CAD build for the part. Positions are in the model's coordinates, mm. A direction names the side the tool comes from. Coordinates: 2 decimals unless noted, no trailing zeros. Loops run counter-clockwise (first coordinate to the right, second up) from the corner with the lowest first, then second, coordinate; pieces in that order, holes last. Notation, with made-up numbers: (43, 33) -> (64, 33) arc R9 cw to (64, 40) -> close; hole circle Ø5 at (32, 78). An arc over 180 degrees is marked (long way). Write each question's results on one line, items separated by ' | '.
Autodesk Inventor part; units mm, degrees
ref_plane "YZ Plane" through (0, 0, 0) normal (1, 0, 0) x (0, 1, 0)
ref_plane "XZ Plane" through (0, 0, 0) normal (0, 1, 0) x (-1, 0, 0)
ref_plane "XY Plane" through (0, 0, 0) normal (0, 0, 1) x (1, 0, 0)
sketch "Boceto1" plane through (0, 0, 0) normal (0, 1, 0) x (-1, 0, 0)
  circle A0 centre (28.5, 0) radius 1.5
  circle A1 centre (28.5, -8) radius 1.5
  circle A2 centre (28.5, 8) radius 1.5
  circle A3 centre (36.5, 0) radius 1.5
  circle A4 centre (20.5, 0) radius 1.5
  circle A5 centre (28.5, 0) radius 47.5
  line L0 (57, 33) -> (43, 33)
  line L1 (43, 33) -> (43, 30)
  line L2 (35.5, 30) -> (35.5, 33)
  line L3 (35.5, 33) -> (21.5, 33)
  line L4 (21.5, 33) -> (21.5, 30)
  line L5 (14, 30) -> (14, 33)
  line L6 (14, 33) -> (0, 33)
  line L7 (43, 30) -> (57, 30)
  line L8 (21.5, 30) -> (35.5, 30)
  line L9 (14, 30) -> (0, 30)
  line L10 (0, 30) -> (0, 33)
  line L11 (57, 33) -> (57, 30)
  line L12 (35.5, -30) -> (35.5, -33)
  line L13 (21.5, -30) -> (35.5, -30)
  line L14 (35.5, -33) -> (21.5, -33)
  line L15 (21.5, -33) -> (21.5, -30)
  line L16 (57, -33) -> (43, -33)
  line L17 (43, -33) -> (43, -30)
  line L18 (43, -30) -> (57, -30)
  line L19 (14, -30) -> (14, -33)
  line L20 (14, -30) -> (0, -30)
  line L21 (14, -33) -> (0, -33)
  line L22 (0, -30) -> (0, -33)
  line L23 (57, -33) -> (57, -30)
extrude "Extrusión1" add sketch "Boceto1" along normal blind 3
sketch "Boceto2" plane through (-28.5, 0, 0) normal (0, -1, 0) x (1, 0, 0)
  circle A0 centre (0, 0) radius 3.5
  point P0 (28.5, 0)
  dimension "d23" = 7
extrude "Extrusión2" cut sketch "Boceto2" against normal blind 10
sketch "Boceto3" plane through (-28.5, 0, 0) normal (0, -1, 0) x (1, 0, 0)
  circle A0 centre (0, 0) radius 4.5
  point P0 (28.5, 0)
  dimension "d26" = 9
extrude "Extrusión3" cut sketch "Boceto3" against normal blind 10
sketch "Boceto4" plane through (-28.5, 0, 0) normal (0, -1, 0) x (1, 0, 0)
  arc A0 (-36.5, 30) -> (-36.5, -30) centre (0, 0) ccw
  line L0 (-28.5, 30) -> (-28.5, 33)
  line L1 (-36.5, 30) -> (-109.5, 30)
  line L2 (-109.5, 30) -> (-109.5, -30)
  line L3 (-28.5, -33) -> (-28.5, -30)
  line L4 (-109.5, -30) -> (-36.5, -30)
extrude "Extrusión4" add sketch "Boceto4" against normal blind 3
sketch "Boceto5" plane through (0, 3, 0) normal (0, 1, 0) x (1, 0, 0)
  line L0 (-11.1092, 17.1983) -> (-42.6801, 17.1983)
  line L1 (-42.6801, 17.1983) -> (-42.6801, -13.2583)
  line L2 (-42.6801, -13.2583) -> (-11.1092, -13.2583)
  line L3 (-11.1092, -13.2583) -> (-11.1092, 17.1983)
  point P0 (0, 0)
extrude "Extrusión5" add sketch "Boceto5" against normal blind 3
properties part number "base3"
Q1. Pull direction X, two halves, no side cores. Call faces 1 (the flat face through (-29, 1, 33)), 2 (the flat face through (-58, 0, 1)), 3 (the cylindrical face through (18.972, 1.479, -1.634)): +X half, -X half, draft (parallel to the pull), parting line (faces both ways), or undercut.
Results are:
face 1: undercut | face 2: draft | face 3: parting line
Q2. Cut at C-C on x = -48. Write the cut outline in (y, z), and give its area (3 significant figures).
Results are:
outline: (0, -43.31) -> (3, -43.31) -> (3, -33) -> (0, -33) -> close; (0, -30) -> (3, -30) -> (3, 30) -> (0, 30) -> close; (0, 33) -> (3, 33) -> (3, 43.31) -> (0, 43.31) -> close | area: 242 mm^2
Q3. Drop flat-ended pins along their axis: pin 1 (0.9 mm diameter, centred on y = 1.5, z = -32, fed in from +X); pin 2 (1.5 mm diameter, centred on y = 1.5, z = 31.5, fed in from -X); pin 3 (1.5 mm diameter, centred on x = -118, y = 1, fed in from +Z). Give the stop position or say it passes through.
Results are:
pin 1: x = 7.01 | pin 2: x = -64.7 | pin 3: z = 30
Q4. Cut at B-B on y = 1.55. Write the cut outline in (x, z).
Results are:
outline: (-138, -30) -> (-65.33, -30) arc R47.5 ccw (long way) to (-65.33, 30) -> (-138, 30) -> close; hole (-57, -33) -> (-43, -33) -> (-43, -30) -> (-57, -30) -> close; hole (-57, 30) -> (-43, 30) -> (-43, 33) -> (-57, 33) -> close; hole (-35.5, -33) -> (-21.5, -33) -> (-21.5, -30) -> (-35.5, -30) -> close; hole (-35.5, 30) -> (-21.5, 30) -> (-21.5, 33) -> (-35.5, 33) -> close; hole (-14, -33) -> (0, -33) -> (0, -30) -> (-14, -30) -> close; hole (-14, 30) -> (0, 30) -> (0, 33) -> (-14, 33) -> close
Q5. Wall check: L1, parallel to Z at x = -27, y = 1.95; L2, parallel to Z at x = -44.5, y = 0.5; L3, parallel to Z at x = -76.5, y = 1.8. Give the ranges that are in metal, low to high. Write a range as from..to.
Results are:
L1: -47.48..-33, -30..30, 33..47.48 | L2: -44.72..-33, -30..30, 33..44.72 | L3: -30..30
Q6. Cut at D-D on x = -105. Write the cut outline in (y, z), and give its area (3 significant figures).
Results are:
outline: (0, -30) -> (3, -30) -> (3, 30) -> (0, 30) -> close | area: 180 mm^2
Q7. Cut at A-A on x = -28.5. Write the cut outline in (y, z).
Results are:
outline: (0, -47.5) -> (3, -47.5) -> (3, -33) -> (0, -33) -> close; (0, -30) -> (3, -30) -> (3, 30) -> (0, 30) -> close; (0, 33) -> (3, 33) -> (3, 47.5) -> (0, 47.5) -> close
Q8. Which spindle directions (+Z, -Z, +X, -X, +Y, -Y) get a long thin tool onto all of the face, cutting with end or side? Do faces 4 (the flat face through (-102, 1, -30)), 5 (the flat face through (-61, 3, 1)), 6 (the flat face through (-50, 1, 30)). Say none if no direction does.
Results are:
face 4: -Z, -X, +Y, -Y | face 5: +Z, -Z, +X, -X, +Y | face 6: +Y, -Y
